from build123d import *

# Parameters (mm, degrees)
EXTRUDE_1_DEPTH     = 4
SKETCH_3_R          = 1.5
EXTRUDE_2_DEPTH     = 6
SKETCH_4_R          = 3
CUT_EXTRUDE_1_DEPTH = 2.5


with BuildPart() as part:
    # ｽｹｯﾁ2 → ﾎﾞｽ - 押し出し1 (new body)
    with BuildSketch(Plane.XY):
        Polygon((3.897114317, -2.25), (3.897114317, 2.25), (0, 4.5), (-3.897114317, 2.25), (-3.897114317, -2.25), (0, -4.5), align=None)
    extrude(amount=EXTRUDE_1_DEPTH)

    # ｽｹｯﾁ3 → ﾎﾞｽ - 押し出し2 (add)
    with BuildSketch(Plane(origin=(0, 0, 0), x_dir=(-1, 0, 0), z_dir=(0, 0, -1))):
        Circle(SKETCH_3_R)
    extrude(amount=EXTRUDE_2_DEPTH)

    # ｽｹｯﾁ4 → ｶｯﾄ - 押し出し1 (cut)
    with BuildSketch(Plane.XY.offset(4)):
        Circle(SKETCH_4_R)
    extrude(amount=-CUT_EXTRUDE_1_DEPTH, mode=Mode.SUBTRACT)


solid = part.part
Design review of the part built by this model. Coordinates are the model's own, in mm. A direction names the side the tool comes from. Round coordinates to 2 decimals unless told otherwise and drop trailing zeros. Write each loop counter-clockwise with the first axis right and the second up, starting at its lowest first coordinate (ties: lowest second). Pieces come first, ordered by that corner, then holes. Notation, with made-up numbers: (77.25, -29) - (92.25, -29) arc R23 cw to (92.25, -9) - close; hole circle Ø3 at (27.5, 60). An arc over 180 degrees is marked (long way). Use a Markdown table: item, result. Add a question column.
1. We need section A-A (z = 3). State the section outline as (x, y) points.
2. Clearance check with flat-ended pins moving along their axes: pin 1 (3 mm diameter, centred on x = 0.5, y = -2.5, fed in from +Z); pin 2 (3 mm diameter, centred on x = 0, y = 0, fed in from +Z). State where each tip first meets the part, or that it passes through.
3. We need section C-C (x = -1.75). State the section outline as (y, z) points.
4. We need section B-B (y = 0). State the section outline as (x, z) points.
5. Mouldability with a two-part tool opening along Y and no side actions: class faces 1 (the face through (0, 0, 1.5)), 2 (the face through (-1.976, -3.359, 1.972)), 3 (the face through (3.897, 0, 2)) as +Y half, -Y half, draft (parallel to the pull), parting line (faces both ways), or undercut.
6. Wall thickness on probe 1 along Z at (x, y) = (1, -2.75); probe 2 along Z at (x, y) = (-1.25, 0.5); probe 3 along X at (y, z) = (-0.25, 3.75): over which ranges is each line inside the solid? List them lowest first.
7. We need section D-D (z = -3.5). State the section outline as (x, y) points, then the cut area to 3 significant figures.
8. For faces 4 (the face through (0, -2, 0)), 5 (the face through (-3, 0, 3)), 6 (the face through (1.92, -3.39, 1.97)), list the 3-axis set-ups (+Z, -Z, +X, -X, +Y, -Y) from which the entire face can be reached by the end or side of a thin tool; tool diameter is ignored.
Output:
| question | item | result |
|---|---|---|
| 1 | outline | (-3.9, -2.25) - (0, -4.5) - (3.9, -2.25) - (3.9, 2.25) - (0, 4.5) - (-3.9, 2.25) - close; hole circle Ø6 at (0, 0) |
| 2 | pin 1 | stops at z = 4 |
| 2 | pin 2 | stops at z = 1.5 |
| 3 | outline | (-3.49, 0) - (3.49, 0) - (3.49, 4) - (2.44, 4) - (2.44, 1.5) - (-2.44, 1.5) - (-2.44, 4) - (-3.49, 4) - close |
| 4 | outline | (-3.9, 0) - (-1.5, 0) - (-1.5, -6) - (1.5, -6) - (1.5, 0) - (3.9, 0) - (3.9, 4) - (3, 4) - (3, 1.5) - (-3, 1.5) - (-3, 4) - (-3.9, 4) - close |
| 5 | face 1 | undercut |
| 5 | face 2 | -Y half |
| 5 | face 3 | draft |
| 6 | probe 1 | z = 0 to 1.5 |
| 6 | probe 2 | z = -6 to 1.5 |
| 6 | probe 3 | x = -3.9 to -2.99, 2.99 to 3.9 |
| 7 | outline | circle Ø3 at (0, 0) |
| 7 | area | 7.07 mm2 |
| 8 | face 4 | -Z |
| 8 | face 5 | +Z |
| 8 | face 6 | +Z, -Z, +X, -Y |
